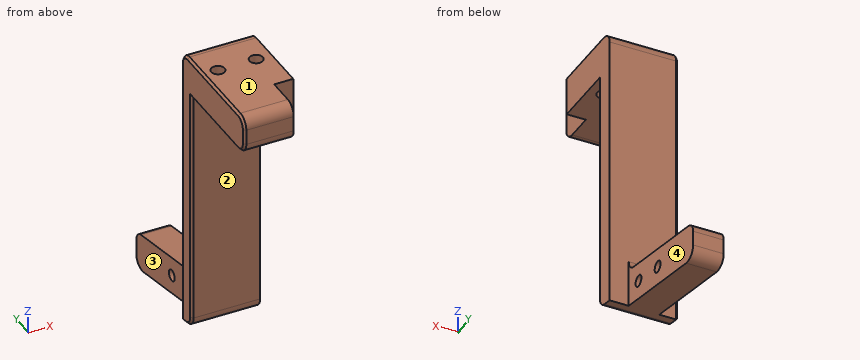
from build123d import *

# Parameters (mm, degrees)
EXTRUDE_1_DEPTH     = 9
CUT_EXTRUDE_1_DEPTH = 5
SKETCH_3_R          = 1.75
CUT_EXTRUDE_2_DEPTH = 50.647599136312735
SKETCH_4_W          = 3.000000000000001
SKETCH_4_H          = 19.851507449534697
EXTRUDE_2_DEPTH     = 5.5
FILLET_2_R          = 5
FILLET_3_R          = 5
SKETCH_6_W          = 18
SKETCH_6_H          = 10.000000000000004
EXTRUDE_3_DEPTH     = 16.2
CUT_EXTRUDE_5_DEPTH = 52.567649463300064
CUT_EXTRUDE_6_DEPTH = 53.49411618001278
EXTRUDE_4_DEPTH     = 18
SKETCH_11_W         = 4.999999999999995
SKETCH_11_H         = 18.60004044786868
CUT_EXTRUDE_7_DEPTH = 33
SKETCH_12_R         = 1.4999999999999973
CUT_EXTRUDE_8_DEPTH = 90.33116605445798
FILLET_4_R          = 3
CHAMFER_3_SIZE      = 0.6


# Some blends are built 0.0001 mm under size
with BuildPart() as part:
    # ｽｹｯﾁ1 → ﾎﾞｽ - 押し出し1 (new, symmetric)
    with BuildSketch(Plane(origin=(0, 0, 0), x_dir=(0, 0, -1), z_dir=(1, 0, 0))):
        Polygon((-5.0000000000000036, -6.499999999999999), (5.0000000000000036, -6.499999999999999), (5.0000000000000036, 6.499999999999999), (13.25805060886326, 47.79), (3.2580506088632593, 47.79), (-5.0000000000000036, 6.500000000000001), align=None)
    extrude(amount=EXTRUDE_1_DEPTH, both=True)

    # ｽｹｯﾁ2 → ｶｯﾄ - 押し出し1 (cut)
    with BuildSketch(Plane(origin=(9, 0, 0), x_dir=(0, 0, -1), z_dir=(1, 0, 0))):
        Polygon((3.2580506088632593, 47.790000000000006), (-1.10677614066039, 25.966000000000005), (8.50860394182422, 24.04291219799919), (13.258050608863256, 47.790000000000006), align=None)
    cut_extrude_1 = extrude(amount=-CUT_EXTRUDE_1_DEPTH, mode=Mode.SUBTRACT)

    # ﾐﾗｰ1: ｶｯﾄ - 押し出し1 across plane
    add(cut_extrude_1.mirror(Plane(origin=(0, 0, 0), x_dir=(0, 0, 1), z_dir=(1, 0, 0))), mode=Mode.SUBTRACT)

    # ｽｹｯﾁ3 → ｶｯﾄ - 押し出し2 (cut, through all)
    with BuildSketch(Plane(origin=(0, 0, -5.0000000000000036), x_dir=(-1, 0, 0), z_dir=(0, 0, -1))):
        with Locations((5, -1.4999999999999987)):
            Circle(SKETCH_3_R)
        with Locations((-5, -1.4999999999999987)):
            Circle(SKETCH_3_R)
    extrude(amount=-CUT_EXTRUDE_2_DEPTH, mode=Mode.SUBTRACT)

    # ｽｹｯﾁ4 → ﾎﾞｽ - 押し出し2 (add)
    with BuildSketch(Plane(origin=(0, 1.2115468473854123, 6.057697112542844), x_dir=(1, 0, 0), z_dir=(0, 0.19611729080206414, 0.980580444557436))):
        with Locations((7.5, 15.318940160380402)):
            Rectangle(SKETCH_4_W, SKETCH_4_H)
        Polygon((-8.99999999999999, 5.393186435613051), (-8.999999999999993, 25.24469388514775), (-5.999999999999994, 25.244693885147754), (-5.9999999999999885, 5.393186435613052), align=None)
    extrude(amount=EXTRUDE_2_DEPTH)

    # ﾌｨﾚｯﾄ2
    # the kernel refuses this fillet: 5 mm, written as the material it takes off along each edge
    with BuildSketch(Plane(origin=(-19.247567109880233, 47.79, -13.25805060886326), x_dir=(0, -0.9805804445574373, 0.19611729080205748), z_dir=(1, 0, 0))) as fillet_2_piece_1:
        with BuildLine():
            CenterArc((FILLET_2_R * 1.21980536879, -FILLET_2_R), FILLET_2_R, 90.00000000000003, 101.30999999999938)
            Line((FILLET_2_R * 0.239224924233, -FILLET_2_R * 1.1961172908), (0, 0))
            Line((0, 0), (FILLET_2_R * 1.21980536879, 2e-17))
        make_face()
    extrude(amount=38.495134219760466, mode=Mode.SUBTRACT)
    with BuildSketch(Plane(origin=(14.247536467555662, 47.79, -3.2580506088632593), x_dir=(0, 0, -1), z_dir=(-1, 0, 0))) as fillet_2_piece_2:
        with BuildLine():
            CenterArc((FILLET_2_R * 0.819802917404, FILLET_2_R), FILLET_2_R, 191.30999999999946, 78.69000000000051)
            Line((-FILLET_2_R * 0.160777527153, FILLET_2_R * 0.803882709198), (0, 0))
            Line((0, 0), (FILLET_2_R * 0.819802917404, 0))
        make_face()
    extrude(amount=28.495072935111324, mode=Mode.SUBTRACT)

    # ﾌｨﾚｯﾄ3
    fillet_3_edges = [part.edges().sort_by_distance(p)[0] for p in [
        (-4, 25.004456098999597, -3.7009139005819147),
        (4, 25.004456098999597, -3.7009139005819147),
    ]]
    fillet(fillet_3_edges, radius=FILLET_3_R - 0.0001)  # a hair under: the kernel refuses the full size

    # 面取り2
    # the kernel refuses this chamfer: 1 mm, written as the material it takes off along each edge
    with BuildSketch(Plane(origin=(9, 23.43957972269821, -11.525247830932894), x_dir=(-0.9850292351397439, 0.16903968557305887, -0.0338081443053687), z_dir=(0, 0.19611729080206025, 0.9805804445574368))) as chamfer_2_piece_1:
        with BuildLine():
            Line((1.2305543745450382, 1e-17), (-0.4179125111005865, 1.157416606835036))
            Line((-0.4179125111005865, 1.157416606835036), (-0.5656668963715484, 1.1315585010807419))
            ThreePointArc((-0.5656668963715484, 1.1315585010807419), (-0.2522325130461084, 0.5711346395907222), (-0.14775438527096194, -0.02585810575429407))
            Line((-0.14775438527096194, -0.02585810575429407), (0.02585810575429378, -0.14775438527096027))
            ThreePointArc((0.02585810575429378, -0.14775438527096027), (0.6228508510993123, -0.04327625749581342), (1.2564124802993322, -0.14775438527096027))
            Line((1.2564124802993322, -0.14775438527096027), (1.2305543745450382, 1e-17))
        make_face()
    extrude(amount=21.458576318299393, mode=Mode.SUBTRACT)

    # ｽｹｯﾁ6 → ﾎﾞｽ - 押し出し3 (add)
    with BuildSketch(Plane.XZ.offset(6.499999999999999)):
        Rectangle(SKETCH_6_W, SKETCH_6_H)
    extrude(amount=EXTRUDE_3_DEPTH)

    # ｽｹｯﾁ7 → ｶｯﾄ - 押し出し5 (cut, through all)
    with BuildSketch(Plane.XY.offset(5.0000000000000036)):
        Polygon((9, -22.7), (3.9999999999999982, -22.7), (3.9999999999999982, -12.700000000000001), (9, -12.7), align=None)
    extrude(amount=-CUT_EXTRUDE_5_DEPTH, mode=Mode.SUBTRACT)

    # ｽｹｯﾁ8 → ｶｯﾄ - 押し出し6 (cut, through all)
    with BuildSketch(Plane(origin=(9, 0, 0), x_dir=(0, 0, -1), z_dir=(1, 0, 0))):
        Polygon((-14.730367070472871, 56.5), (-14.730367070472871, 6.499999999999999), (-5.0000000000000036, 6.499999999999999), (-10.393192445065868, 7.578645099411347), (-6.696085876528205, 26.064064654853848), (8.31248665102216, 23.062331753441747), (5.0000000000000036, 6.499999999999999), (15.269632929527129, 6.499999999999999), (15.269632929527127, 56.5), align=None)
        Polygon((-10.393192445065868, 7.578645099411347), (-5.0000000000000036, 6.500000000000001), (5.000000000000002, 6.499999999999999), (8.31248665102216, 23.062331753441747), (-6.696085876528205, 26.064064654853848), align=None)
    extrude(amount=-CUT_EXTRUDE_6_DEPTH, mode=Mode.SUBTRACT)

    # ｽｹｯﾁ10 → ﾎﾞｽ - 押し出し4 (add)
    with BuildSketch(Plane(origin=(9, 0, 0), x_dir=(0, 0, -1), z_dir=(1, 0, 0))):
        Polygon((61.000006128464946, 9.300000000000002), (-5.0000000000000036, 9.300000000000002), (-5.0000000000000036, 6.499999999999999), (5.000000000000002, 6.499999999999999), (5.0000000000000036, 4.299999999999994), (69.99999999999999, 4.300000000000002), (77.60004657633361, 42.300000000000004), (67.60004657633361, 42.3), align=None)
    extrude(amount=-EXTRUDE_4_DEPTH)

    # ｽｹｯﾁ11 → ｶｯﾄ - 押し出し7 (cut)
    with BuildSketch(Plane(origin=(0, 42.29999999999995, 2.935e-14), x_dir=(1, 0, 0), z_dir=(0, 1, 0))):
        with Locations((-6.499999999999997, 68.30002635239924)):
            Rectangle(SKETCH_11_W, SKETCH_11_H)
        Polygon((4, 77.60004657633358), (4, 59.0000061284649), (8.999999999999995, 59.0000061284649), (9, 77.60004657633358), align=None)
    extrude(amount=-CUT_EXTRUDE_7_DEPTH, mode=Mode.SUBTRACT)

    # ｽｹｯﾁ12 → ｶｯﾄ - 押し出し8 (cut, through all)
    with BuildSketch(Plane(origin=(4, 0, 0), x_dir=(-5e-17, 0, -1), z_dir=(1, 0, -5e-17))):
        with Locations((68.96118516495055, 24.105804445574364)):
            Circle(SKETCH_12_R)
        with Locations((67.00001225692989, 14.300000000000004)):
            Circle(SKETCH_12_R)
    extrude(amount=-CUT_EXTRUDE_8_DEPTH, mode=Mode.SUBTRACT)

    # ﾌｨﾚｯﾄ4
    fillet_4_edges = [part.edges().sort_by_distance(p)[0] for p in [
        (-2.500000000000001, -22.7, -5.000000000000002),
        (-2.5, -22.7, 5.000000000000002),
        (0, 9.300000000000002, 5.0000000000000036),
        (0, 4.3000000000000025, -69.99999999999999),
        (0, 42.300000000000004, -77.60004657633361),
        (0, 42.3, -67.60004657633361),
        (0, 9.300000000000002, -61.000006128464946),
    ]]
    fillet(fillet_4_edges, radius=FILLET_4_R)

    # 面取り3
    chamfer_3_edges = [part.edges().sort_by_distance(p)[0] for p in [
        (-8.999999999999998, 9.299999999999974, -34.50000306423246),
        (-9, 4.299999999999998, -36.27029562389333),
        (-9, -22.7, 0),
        (-9, 8.005824063796883, -70.74116935496194),
        (-9, -7.700000000000004, -5.000000000000003),
        (-9, -6.699999999999992, 5.000000000000003),
        (-9, 8.421320343559644, 4.1213203435596455),
        (-9, 4.979972455204619, -69.4425565974686),
        (-9, -21.821320343559645, -4.1213203435596455),
        (-9, -21.82132034355964, 4.1213203435596455),
    ]]
    chamfer(chamfer_3_edges, length=CHAMFER_3_SIZE)


solid = part.part
The listing builds one solid part. Answer for the finished solid, in the listing's coordinates (mm). Face numbers are marked on the shaded views. A direction names the side the tool comes from. Coordinates: 2 decimals unless noted, no trailing zeros. Write each loop counter-clockwise with the first axis right and the second up, starting at its lowest first coordinate (ties: lowest second). Pieces come first, ordered by that corner, then holes. Notation, with made-up numbers: (88.5, 44) - (117.5, 44) arc R5 ccw to (117.5, 48) - close; hole circle Ø11 at (54, 49). An arc over 180 degrees is marked (long way). Return JSON: item names as keys, results as strings.
1. Which of the six approach directions +Z, -Z, +X, -X, +Y, -Y give full straight-line access (tool end or side, diameter ignored) to the marked faces 1, 2, 3 and 4?
Final values:
{"face 1": "+Z, +X, -X, +Y, -Y", "face 2": "-Z, +X, -X, -Y", "face 3": "+Z, -Z, -X, +Y", "face 4": "+Z, -Z, +X, +Y"}
2. Consider line 1 along X through (y, z) = (-1, -2); line 2 along Y through (x, z) = (1.75, -1.5); line 3 along X through (y, z) = (-13.5, -2). Determine where each line is inside the solid, lowest interval first.
Final values:
{"line 1": "-9 to -6.68, -3.32 to 3.32, 6.68 to 9", "line 2": "-22.7 to 9.3", "line 3": "-9 to 4"}
3. The part is cut by section A-A on x = 5. Determine the outline of the cut face in (y, z), then the cut area to 3 significant figures.
Final values:
{"outline": "(-12.7, -5) - (-3.25, -5) - (-3.25, 5) - (-12.7, 5) - close; (0.25, -5) - (4.3, -5) - (4.3, -67.54) arc R3 ccw to (6.71, -70.48) - (9.3, -71) - (9.3, 2) arc R3 ccw to (6.3, 5) - (0.25, 5) - close", "area": "509 mm^2"}
4. Each of these flat-tipped pins is pushed along its axis until it touches: pin 1 Ø5 at (x, z) = (5, -56.5) entering from +Y; pin 2 Ø5 at (y, z) = (-18.5, -1.5) entering from +X; pin 3 Ø6 at (x, z) = (4, -37.5) entering from -Y. Where does it stop, or does it pass through?
Final values:
{"pin 1": "y = 9.31", "pin 2": "x = 4", "pin 3": "y = 4.3"}
5. The part is cut by section B-B on y = -1.5. Determine the outline of the cut face in (x, z).
Final values:
{"outline": "(-9, -4.4) - (-8.4, -5) - (-6.75, -5) - (-6.75, 5) - (-8.4, 5) - (-9, 4.4) - close; (-3.25, -5) - (3.25, -5) - (3.25, 5) - (-3.25, 5) - close; (6.75, -5) - (9, -5) - (9, 5) - (6.75, 5) - close"}
6. The part is cut by section D-D on y = 14.3. Determine the outline of the cut face in (x, z), then the cut area to 3 significant figures.
Final values:
{"outline": "(-4, -72) - (4, -72) - (4, -68.5) - (-4, -68.5) - close; (-4, -65.5) - (4, -65.5) - (4, -62) - (-4, -62) - close", "area": "56.0 mm^2"}
7. The part is cut by section C-C on x = -5. Determine the outline of the cut face in (y, z), then the cut area to 3 significant figures.
Final values:
{"outline": "(-22.7, -2) arc R3 ccw to (-19.7, -5) - (-3.25, -5) - (-3.25, 5) - (-19.7, 5) arc R3 ccw to (-22.7, 2) - close; (0.25, -5) - (4.3, -5) - (4.3, -67.54) arc R3 ccw to (6.71, -70.48) - (9.3, -71) - (9.3, 2) arc R3 ccw to (6.3, 5) - (0.25, 5) - close", "area": "606 mm^2"}
